```python
from build123d import *

# Parameters (mm, degrees)
SKETCH1_R           = 6
BOSS_EXTRUDE1_DEPTH = 20


with BuildPart() as part:
    # Sketch1 → Boss-Extrude1 (new body)
    with BuildSketch(Plane(origin=(0, 0, 0), x_dir=(1, 0, 0), z_dir=(0, 1, 0))):
        with BuildLine():
            ThreePointArc((40, 69.282032303), (-80, 0), (40, -69.282032303))
            ThreePointArc((40, -69.282032303), (60, -63.923048454), (80, -69.282032303))
            ThreePointArc((80, -69.282032303), (200, 0), (80, 69.282032303))
            ThreePointArc((80, 69.282032303), (60, 63.923048454), (40, 69.282032303))
        make_face()
        Circle(SKETCH1_R, mode=Mode.SUBTRACT)
        with Locations((120, 0)):
            Circle(SKETCH1_R, mode=Mode.SUBTRACT)
        with BuildLine():
            Line((55, 20), (55, 49.839779322))
            ThreePointArc((55, 49.839779322), (53.843530574, 53.037790068), (50.909090909, 54.756440152))
            ThreePointArc((50.909090909, 54.756440152), (42.704102554, 57.009810114), (35, 60.621778265))
            ThreePointArc((35, 60.621778265), (-3.755089291, 69.899208182), (-41.293201923, 56.523194133))
            ThreePointArc((-41.293201923, 56.523194133), (-43.328783805, 52.871588373), (-41.879221406, 48.950289217))
            Line((-41.879221406, 48.950289217), (-6.464466094, 13.535533906))
            ThreePointArc((-6.464466094, 13.535533906), (-3.31413574, 14.629302933), (0, 15))
            Line((0, 15), (50, 15))
            ThreePointArc((50, 15), (53.535533906, 16.464466094), (55, 20))
        make_face(mode=Mode.SUBTRACT)
        with BuildLine():
            Line((0, -15), (50, -15))
            ThreePointArc((50, -15), (53.535533906, -16.464466094), (55, -20))
            Line((55, -20), (55, -49.839779322))
            ThreePointArc((55, -49.839779322), (53.843530574, -53.037790068), (50.909090909, -54.756440152))
            ThreePointArc((50.909090909, -54.756440152), (42.704102554, -57.009810114), (35, -60.621778265))
            ThreePointArc((35, -60.621778265), (-3.755089291, -69.899208182), (-41.293201923, -56.523194133))
            ThreePointArc((-41.293201923, -56.523194133), (-43.328783805, -52.871588373), (-41.879221406, -48.950289217))
            Line((-41.879221406, -48.950289217), (-6.464466094, -13.535533906))
            ThreePointArc((-6.464466094, -13.535533906), (-3.31413574, -14.629302933), (0, -15))
        make_face(mode=Mode.SUBTRACT)
        with BuildLine():
            Line((65, 20), (65, 49.839779322))
            ThreePointArc((65, 49.839779322), (66.156469426, 53.037790068), (69.090909091, 54.756440152))
            ThreePointArc((69.090909091, 54.756440152), (77.295897446, 57.009810114), (85, 60.621778265))
            ThreePointArc((85, 60.621778265), (123.755089291, 69.899208182), (161.293201923, 56.523194133))
            ThreePointArc((161.293201923, 56.523194133), (163.328783805, 52.871588373), (161.879221406, 48.950289217))
            Line((161.879221406, 48.950289217), (126.464466094, 13.535533906))
            ThreePointArc((126.464466094, 13.535533906), (123.31413574, 14.629302933), (120, 15))
            Line((120, 15), (70, 15))
            ThreePointArc((70, 15), (66.464466094, 16.464466094), (65, 20))
        make_face(mode=Mode.SUBTRACT)
        with BuildLine():
            Line((65, -20), (65, -49.839779322))
            ThreePointArc((65, -49.839779322), (66.156469426, -53.037790068), (69.090909091, -54.756440152))
            ThreePointArc((69.090909091, -54.756440152), (77.295897446, -57.009810114), (85, -60.621778265))
            ThreePointArc((85, -60.621778265), (123.755089291, -69.899208182), (161.293201923, -56.523194133))
            ThreePointArc((161.293201923, -56.523194133), (163.328783805, -52.871588373), (161.879221406, -48.950289217))
            Line((161.879221406, -48.950289217), (126.464466094, -13.535533906))
            ThreePointArc((126.464466094, -13.535533906), (123.31413574, -14.629302933), (120, -15))
            Line((120, -15), (70, -15))
            ThreePointArc((70, -15), (66.464466094, -16.464466094), (65, -20))
        make_face(mode=Mode.SUBTRACT)
        with BuildLine():
            Line((134.142135624, 5), (184.226162893, 5))
            ThreePointArc((184.226162893, 5), (188.02393552, 6.747781822), (189.166636962, 10.769230769))
            ThreePointArc((189.166636962, 10.769230769), (184.671567276, 26.787840266), (176.523194133, 41.293201923))
            ThreePointArc((176.523194133, 41.293201923), (172.871588373, 43.328783805), (168.950289217, 41.879221406))
            Line((168.950289217, 41.879221406), (133.535533906, 6.464466094))
            ThreePointArc((133.535533906, 6.464466094), (133.858192988, 5.740251485), (134.142135624, 5))
        make_face(mode=Mode.SUBTRACT)
        with BuildLine():
            Line((134.142135624, -5), (184.226162893, -5))
            ThreePointArc((184.226162893, -5), (188.02393552, -6.747781822), (189.166636962, -10.769230769))
            ThreePointArc((189.166636962, -10.769230769), (184.671567276, -26.787840266), (176.523194133, -41.293201923))
            ThreePointArc((176.523194133, -41.293201923), (172.871588373, -43.328783805), (168.950289217, -41.879221406))
            Line((168.950289217, -41.879221406), (133.535533906, -6.464466094))
            ThreePointArc((133.535533906, -6.464466094), (133.858192988, -5.740251485), (134.142135624, -5))
        make_face(mode=Mode.SUBTRACT)
        with BuildLine():
            Line((-13.535533906, 6.464466094), (-48.950289217, 41.879221406))
            ThreePointArc((-48.950289217, 41.879221406), (-52.871588373, 43.328783805), (-56.523194133, 41.293201923))
            ThreePointArc((-56.523194133, 41.293201923), (-64.671567276, 26.787840266), (-69.166636962, 10.769230769))
            ThreePointArc((-69.166636962, 10.769230769), (-68.02393552, 6.747781822), (-64.226162893, 5))
            Line((-64.226162893, 5), (-14.142135624, 5))
            ThreePointArc((-14.142135624, 5), (-13.858192988, 5.740251485), (-13.535533906, 6.464466094))
        make_face(mode=Mode.SUBTRACT)
        with BuildLine():
            Line((-14.142135624, -5), (-64.226162893, -5))
            ThreePointArc((-64.226162893, -5), (-68.02393552, -6.747781822), (-69.166636962, -10.769230769))
            ThreePointArc((-69.166636962, -10.769230769), (-64.671567276, -26.787840266), (-56.523194133, -41.293201923))
            ThreePointArc((-56.523194133, -41.293201923), (-52.871588373, -43.328783805), (-48.950289217, -41.879221406))
            Line((-48.950289217, -41.879221406), (-13.535533906, -6.464466094))
            ThreePointArc((-13.535533906, -6.464466094), (-13.858192988, -5.740251485), (-14.142135624, -5))
        make_face(mode=Mode.SUBTRACT)
    extrude(amount=BOSS_EXTRUDE1_DEPTH)


solid = part.part
```
Could you check a few things on this model? Use its own coordinates, in mm. A direction names the side the tool comes from. Coordinates: 2 decimals unless noted, no trailing zeros. Order: outer loops, then holes, each group sorted by start corner. A loop starts at its lowest first (then second) coordinate and runs counter-clockwise, first axis right, second up. Notation, with made-up numbers: M 35.25,32 L 76.25,32 A17 ccw 76.25,63 Z; hole C 84,7 d9. An arc over 180 degrees is marked long. Use a Markdown table: item, result. Add a question column.
Q1. I want a section at D-D on y = 6. Give the number of separate pieces and of enclosed holes in the cut face, then the cut area to 3 significant figures.
Q2. I want a section at B-B on x = 141. List the corners of the cut face in (y, z) for me.
Q3. I'm going to push flat-ended pins straight in: pin 1 (6 mm diameter, centred on x = 82.5, y = 7.5, fed in from +Z); pin 2 (10 mm diameter, centred on y = 5, z = 38, fed in from +X); pin 3 (8 mm diameter, centred on x = 163.5, y = 7.5, fed in from -Z). Where does each tip first touch, or does it pass through?
Q4. I want a section at C-C on x = 90. List the corners of the cut face in (y, z) for me, then the cut area to 3 significant figures.
Q5. If I drill on L1, parallel to Z at x = 120, y = 13.25; L2, parallel to Z at x = 75.5, y = 2.75; L3, parallel to X at y = 12.5, z = -34, over which ranges is the centre line in solid material (lowest first)?
Q6. Which directions (+Z, -Z, +X, -X, +Y, -Y) give clear straight access to the entire face, cutting with the end or side of a thin tool? Please do faces 1 (the flat face through (-39, 10, 5)), 2 (the cylindrical face through (60.293, 9.86, -63.924)).
Q7. I want a section at A-A on z = 0. List the corners of the cut face in (x, y) for me.
Checked values:
| question | item | result |
|---|---|---|
| 1 | separate pieces | 1 |
| 1 | enclosed holes | 10 |
| 1 | area | 15,500 mm² |
| 2 | outline | M 0,-77.19 L 20,-77.19 L 20,-66.78 L 0,-66.78 Z; M 0,-28.07 L 20,-28.07 L 20,-13.93 L 0,-13.93 Z; M 0,-5 L 20,-5 L 20,5 L 0,5 Z; M 0,13.93 L 20,13.93 L 20,28.07 L 0,28.07 Z; M 0,66.78 L 20,66.78 L 20,77.19 L 0,77.19 Z |
| 3 | pin 1 | z = 72.18 |
| 3 | pin 2 | x = 192.88 |
| 3 | pin 3 | z = -69.57 |
| 4 | outline | M 0,-74.16 L 20,-74.16 L 20,-63.25 L 0,-63.25 Z; M 0,-15 L 20,-15 L 20,15 L 0,15 Z; M 0,63.25 L 20,63.25 L 20,74.16 L 0,74.16 Z |
| 4 | area | 1,040 mm² |
| 5 | L1 | -80 to -70, -15 to -6, 6 to 15, 70 to 80 |
| 5 | L2 | -67.05 to -56.39, -15 to 15, 56.39 to 67.05 |
| 5 | L3 | -72.42 to -61.19, -41.07 to -26.93, 55 to 65, 146.93 to 161.07, 181.19 to 192.42 |
| 6 | face 1 | +Y, -Y |
| 6 | face 2 | -Z, +Y, -Y |
| 7 | outline | M -80,0 L -6,0 L -6,20 L -80,20 Z; M 6,0 L 114,0 L 114,20 L 6,20 Z; M 126,0 L 200,0 L 200,20 L 126,20 Z |
